Build history of the part. All positions in model axes, mm. A direction names the side the tool comes from. Coordinates: 2 decimals unless noted, no trailing zeros. Write each loop counter-clockwise with the first axis right and the second up, starting at its lowest first coordinate (ties: lowest second). Pieces come first, ordered by that corner, then holes.
```python
from build123d import *

# Parameters (mm, degrees)
SM_BASE_FLANGE_2_DEPTH = 28
SKETCH_15_W            = 61
SKETCH_15_H            = 46
EXTRUDE_1_DEPTH        = 12
SKETCH_18_W            = 21
SKETCH_18_H            = 2.5
SKETCH_18_W_2          = 42
SKETCH_18_H_2          = 41
CUT_EXTRUDE_1_DEPTH    = 20
SKETCH_19_R            = 1
CUT_EXTRUDE_2_DEPTH    = 69.163406605
SKETCH_20_W            = 21
SKETCH_20_H            = 34
CUT_EXTRUDE_3_DEPTH    = 4
EXTRUDE_2_DEPTH        = 3
PATTERN_LINEAR_1_COUNT = 2
PATTERN_LINEAR_1_PITCH = 58
SKETCH_23_R            = 1.45
SKETCH_23_R_2          = 1.7
CUT_EXTRUDE_4_DEPTH    = 82.792420187
SKETCH_24_R            = 1
SKETCH_24_R_2          = 0.99
CUT_EXTRUDE_5_DEPTH    = 69.163406605
EXTRUDE_3_DEPTH        = 4
PATTERN_LINEAR_2_COUNT = 2
PATTERN_LINEAR_2_PITCH = 50


# Sheet-metal steps are written as plain solids
with BuildPart() as part:
    # 草图1 → 基体-法兰2 (new body)
    with BuildSketch(Plane.XY):
        with BuildLine():
            Line((-27.5, -30), (-27.5, 23))
            ThreePointArc((-27.5, 23), (-26.914213562, 24.414213562), (-25.5, 25))
            Line((-25.5, 25), (25.5, 25))
            ThreePointArc((25.5, 25), (26.914213562, 24.414213562), (27.5, 23))
            Line((27.5, 23), (27.5, -30))
            Line((27.5, -30), (30.5, -30))
            Line((30.5, -30), (30.5, 23))
            ThreePointArc((30.5, 23), (29.035533906, 26.535533906), (25.5, 28))
            Line((25.5, 28), (-25.5, 28))
            ThreePointArc((-25.5, 28), (-29.035533906, 26.535533906), (-30.5, 23))
            Line((-30.5, 23), (-30.5, -30))
            Line((-30.5, -30), (-27.5, -30))
        make_face()
    extrude(amount=SM_BASE_FLANGE_2_DEPTH)

    # 草图15 → 凸台-拉伸1 (add, symmetric)
    with BuildSketch(Plane(origin=(0, 28, 0), x_dir=(1, 0, 0), z_dir=(0, 1, 0))):
        with Locations((0, -14)):
            Rectangle(SKETCH_15_W, SKETCH_15_H)
    extrude(amount=EXTRUDE_1_DEPTH, both=True)

    # 草图18 → 切除-拉伸1 (cut)
    with BuildSketch(Plane.XZ.offset(-16)):
        with Locations((-10.5, 35.75)):
            Rectangle(SKETCH_18_W, SKETCH_18_H)
        with Locations((0, 14)):
            Rectangle(SKETCH_18_W_2, SKETCH_18_H_2)
        with Locations((-10.5, -7.75)):
            Rectangle(SKETCH_18_W, SKETCH_18_H)
    extrude(amount=-CUT_EXTRUDE_1_DEPTH, mode=Mode.SUBTRACT)

    # 草图19 → 切除-拉伸2 (cut, through all)
    with BuildSketch(Plane.XY.offset(37)):
        with Locations((3, 18.5)):
            Circle(SKETCH_19_R)
        with Locations(Location((18, 18.5, 0), (0, 0, 180))):
            Circle(SKETCH_19_R)
        with Locations((18, 33.5)):
            Circle(SKETCH_19_R)
        with Locations(Location((3, 33.5, 0), (0, 0, 180))):
            Circle(SKETCH_19_R)
    extrude(amount=-CUT_EXTRUDE_2_DEPTH, mode=Mode.SUBTRACT)

    # 草图20 → 切除-拉伸3 (cut)
    with BuildSketch(Plane.XZ.offset(-36)):
        with Locations((0, 14)):
            Rectangle(SKETCH_20_W, SKETCH_20_H)
    extrude(amount=-CUT_EXTRUDE_3_DEPTH, mode=Mode.SUBTRACT)

    # 草图21 → 凸台-拉伸2 (add)
    with BuildSketch(Plane.ZY.offset(30.5)):
        Polygon((0, 16), (-9, 16), (0, -20), align=None)
        Polygon((28, 16), (28, -20), (37, 16), align=None)
    extrude_2 = extrude(amount=-EXTRUDE_2_DEPTH)

    # 阵列(线性)1: 凸台-拉伸2 ×2
    with Locations(*[(i * PATTERN_LINEAR_1_PITCH, 0, 0) for i in range(1, PATTERN_LINEAR_1_COUNT)]):
        add(extrude_2)

    # 草图23 → 切除-拉伸4 (cut, through all)
    with BuildSketch(Plane.ZY.offset(30.5)):
        with Locations(Location((14, -13, 0), (0, 0, 270))):
            Circle(SKETCH_23_R)
        with Locations(Location((7, -20, 0), (0, 0, 270))):
            Circle(SKETCH_23_R)
        with Locations(Location((14, -20, 0), (0, 0, 270))):
            Circle(SKETCH_23_R_2)
        with Locations(Location((21, -20, 0), (0, 0, 270))):
            Circle(SKETCH_23_R)
        with Locations(Location((14, -27, 0), (0, 0, 270))):
            Circle(SKETCH_23_R)
        with BuildLine():
            Line((0, -30), (14, -30))
            ThreePointArc((14, -30), (5.397674733, -27.243255374), (0, -20))
            Line((0, -20), (0, -30))
        make_face()
        with BuildLine():
            Line((14, -30), (28, -30))
            Line((28, -30), (28, -20))
            ThreePointArc((28, -20), (22.602325267, -27.243255374), (14, -30))
        make_face()
    extrude(amount=-CUT_EXTRUDE_4_DEPTH, mode=Mode.SUBTRACT)

    # 草图24 → 切除-拉伸5 (cut, through all)
    with BuildSketch(Plane(origin=(0, 0, -9), x_dir=(-1, 0, 0), z_dir=(0, 0, -1))):
        with Locations((-17.52, 26)):
            Circle(SKETCH_24_R)
        with Locations((-10.52, 19)):
            Circle(SKETCH_24_R)
        with Locations((-10.52, 33)):
            Circle(SKETCH_24_R_2)
    extrude(amount=-CUT_EXTRUDE_5_DEPTH, mode=Mode.SUBTRACT)

    # 草图25 → 凸台-拉伸3 (add)
    with BuildSketch(Plane(origin=(0, 0, -9), x_dir=(-1, 0, 0), z_dir=(0, 0, -1))):
        Polygon((30.5, 28.892731946), (21, 20.141290546), (21, 16), (27.5, 16), (30.5, 16), align=None)
    extrude_3 = extrude(amount=EXTRUDE_3_DEPTH)

    # 阵列(线性)2: 凸台-拉伸3 ×2
    with Locations(*[(0, 0, i * PATTERN_LINEAR_2_PITCH) for i in range(1, PATTERN_LINEAR_2_COUNT)]):
        add(extrude_3)


solid = part.part
```
1. Mould opens along Z. For faces 5 (the face through (18.217, 19.476, -7.733)), 6 (the face through (-29.021, -21.339, 20.445)), 7 (the face through (6, 31, 37)) say: +Z half, -Z half, draft (parallel to the pull), parting line (faces both ways), or undercut.
Computed values:
face 5: draft
face 6: undercut
face 7: +Z half
2. Saw through at C-C on z = 35.5. List the corners of the cut face in (x, y).
Computed values:
outline: (-30.5, 10) - (-27.5, 10) - (-27.5, 16) - (-21, 16) - (-21, 36) - (0, 36) - (0, 16) - (27.5, 16) - (27.5, 10) - (30.5, 10) - (30.5, 40) - (-30.5, 40) - close; hole circle Ø2 at (3, 18.5); hole circle Ø2 at (3, 33.5); hole circle Ø2 at (10.52, 19); hole circle Ø1.98 at (10.52, 33); hole circle Ø2 at (17.52, 26); hole circle Ø2 at (18, 18.5); hole circle Ø2 at (18, 33.5)
3. Flat gauge pins, fed straight in: pin 1 (12.5 mm diameter, centred on x = 5, z = 21, fed in from -Y); pin 2 (16 mm diameter, centred on x = 8, y = 28.5, fed in from -Z); pin 3 (22 mm diameter, centred on x = 9.5, y = 24, fed in from +Z). Where does each tip first touch, or does it go through?
Computed values:
pin 1: stops at y = 36
pin 2: stops at z = -9
pin 3: stops at z = 37
4. Saw through at D-D on y = -6.5. List the corners of the cut face in (x, z) (3 decimals).
Computed values:
outline: (-30.5, -3.375) - (-27.5, -3.375) - (-27.5, 31.375) - (-30.5, 31.375) - close; (27.5, -3.375) - (30.5, -3.375) - (30.5, 31.375) - (27.5, 31.375) - close
5. Saw through at A-A on x = -2.5. List the corners of the cut face in (y, z), plus the area to 3 significant figures.
Computed values:
outline: (36, -9) - (40, -9) - (40, -3) - (36, -3) - close; (36, 31) - (40, 31) - (40, 37) - (36, 37) - close
area: 48.0 mm2
6. Probe line 1 along Y through (x, z) = (3, 35.5); line 2 along X through (y, z) = (2, 18); line 3 along Z through (x, y) = (28, -20). List the from-to ranges inside material, lowest first.
Computed values:
line 1: y = 16 to 17.5, 19.5 to 32.5, 34.5 to 40
line 2: x = -30.5 to -27.5, 27.5 to 30.5
line 3: z = 0 to 5.55, 8.45 to 12.3, 15.7 to 19.55, 22.45 to 28
7. 3-axis set-ups, long thin cutter, end or side, ignore diameter. For faces 1 (the face through (0, 38, 31)), 2 (the face through (21, 26, 14)), 3 (the face through (0, 26, -8)), 4 (the face through (-25.82, 24.58, 39.03)): which of +Z, -Z, +X, -X, +Y, -Y reach the whole face in a straight line?
Computed values:
face 1: +Y, -Y
face 2: -Y
face 3: +Z, -Z, -Y
face 4: +Z, +X, +Y
8. Saw through at B-B on y = 31. List the corners of the cut face in (x, z), plus the area to 3 significant figures.
Computed values:
outline: (-30.5, -9) - (-21, -9) - (-21, 37) - (-30.5, 37) - close; (0, -9) - (30.5, -9) - (30.5, 37) - (0, 37) - (0, 34.5) - (21, 34.5) - (21, -6.5) - (0, -6.5) - close
area: 979 mm2
